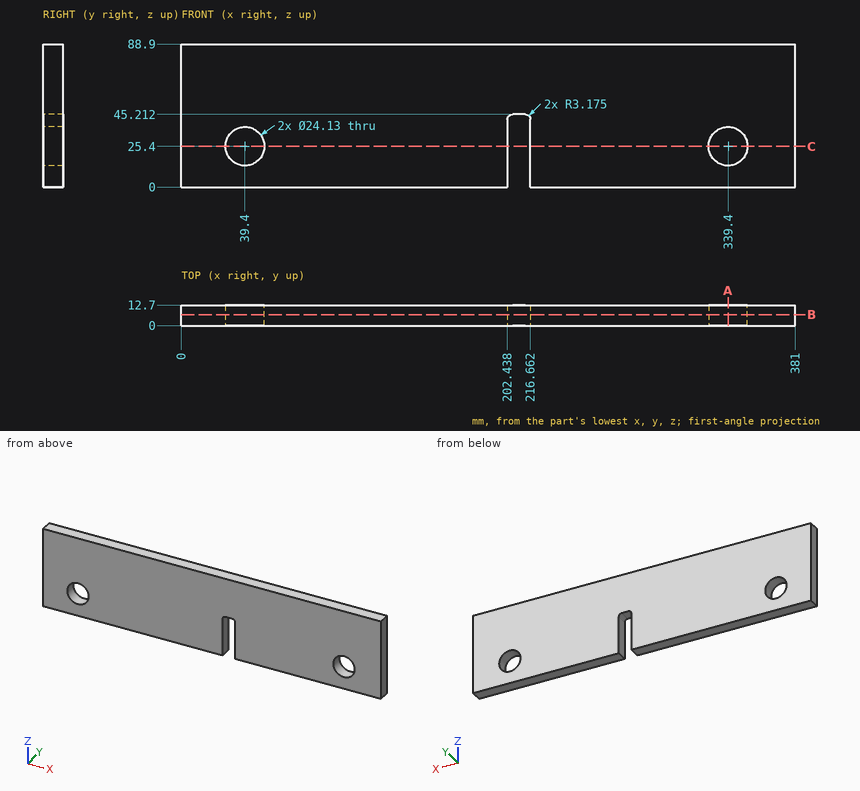
The figure shows three views and two pictorial views of one solid part (mm, origin at its lowest corner). Answer the questions. Coordinates: 2 decimals unless noted, no trailing zeros. Loops run counter-clockwise (first coordinate to the right, second up) from the corner with the lowest first, then second, coordinate; pieces in that order, holes last. Notation, with made-up numbers: (37.25, -14) - (75.25, -14) arc R14 cw to (75.25, 1) - close; hole circle Ø2 at (-29, 19). An arc over 180 degrees is marked (long way). Write item = value, one per line.
1) Find the intervals of material crossed by line 1 along Z through (x, y) = (339.4, 7.75) (3 decimals); line 2 along X through (y, z) = (11.25, 15); line 3 along X through (y, z) = (5.75, 16), in increasing order.
Responses:
line_1 = 0 to 13.335, 37.465 to 88.9
line_2 = 0 to 33.28, 45.52 to 202.44, 216.66 to 333.28, 345.52 to 381
line_3 = 0 to 31.84, 46.96 to 202.44, 216.66 to 331.84, 346.96 to 381
2) Each of these flat-tipped pins is pushed along its axis until it touches: P1, Ø6.5, axis at x = 210, y = 5, coming from the -Z side; P2, Ø21.5, axis at x = 339.4, z = 25.4, coming from the +Y side. Where does it stop, or does it pass through?
Responses:
P1 = 45.21
P2 = through
3) Section A-A (x = 339.4) is taken. Determine the outline of the cut face in (y, z) (3 decimals), plus the area to 3 significant figures.
Responses:
outline = (0, 0) - (12.7, 0) - (12.7, 13.335) - (0, 13.335) - close; (0, 37.465) - (12.7, 37.465) - (12.7, 88.9) - (0, 88.9) - close
area = 823 mm^2
4) Section B-B (y = 6.75) is taken. Determine the outline of the cut face in (x, z) (3 decimals), plus the area to 3 significant figures.
Responses:
outline = (0, 0) - (202.438, 0) - (202.438, 42.037) arc R3.175 cw to (205.613, 45.212) - (213.487, 45.212) arc R3.175 cw to (216.662, 42.037) - (216.662, 0) - (381, 0) - (381, 88.9) - (0, 88.9) - close; hole circle Ø24.13 at (39.4, 25.4); hole circle Ø24.13 at (339.4, 25.4)
area = 32,300 mm^2
5) Section C-C (z = 25.4) is taken. Determine the outline of the cut face in (x, y) (3 decimals), plus the area to 3 significant figures.
Responses:
outline = (0, 0) - (27.335, 0) - (27.335, 12.7) - (0, 12.7) - close; (51.465, 0) - (202.438, 0) - (202.438, 12.7) - (51.465, 12.7) - close; (216.662, 0) - (327.335, 0) - (327.335, 12.7) - (216.662, 12.7) - close; (351.465, 0) - (381, 0) - (381, 12.7) - (351.465, 12.7) - close
area = 4,050 mm^2
